Verification items for this drawing (mm, ordinates from the low corner). A direction names the side the tool comes from. Round coordinates to 2 decimals unless told otherwise and drop trailing zeros. Loops run counter-clockwise (first coordinate to the right, second up) from the corner with the lowest first, then second, coordinate; pieces in that order, holes last. Notation, with made-up numbers: M 34.25,-33 L 92.25,-33 A17 ccw 92.25,-24 Z; hole C 47,18.5 d10. An arc over 180 degrees is marked long. Use one line per item in the form item = value. Start each with the question number.
1. Draft check along Z on the marked faces 1, 2 and 3. Enter one of: pulls with the +Z half, pulls with the -Z half, needs draft (parallel to the pull), parting line crosses it, or undercut.
2. Cross-section at C-C (z = 5). Record the boundary of the cut face in (x, y).
3. Cross-section at D-D (x = 44.65). Record the boundary of the cut face in (y, z), then the cut area to 3 significant figures.
4. Go/stop test with flat-tipped pins: pin 1 (4 mm diameter, centred on x = 39, y = 20, fed in from +Z); pin 2 (10 mm diameter, centred on x = 25.5, y = 16.5, fed in from -Z); pin 3 (3 mm diameter, centred on x = 44.65, y = 15, fed in from +Z); pin 4 (2 mm diameter, centred on x = 5, z = 5, fed in from -Y). Record where each tip stops, or that it passes through.
5. Set-up check for the marked faces 4, 5 and 6: record each of +Z, -Z, +X, -X, +Y, -Y from which the full face is reachable in a straight line by a thin tool's end or side.
6. Cross-section at A-A (y = 15). Record the boundary of the cut face in (x, z), then the cut area to 3 significant figures.
7. Material ranges on line 1 (Y direction, x = 44.65, z = 48.1); line 2 (X direction, y = 3.4, z = 5); line 3 (Y direction, x = 44, z = 48), recorded low to high.
8. Cross-section at B-B (x = 53). Record the boundary of the cut face in (y, z), then the cut area to 3 significant figures.
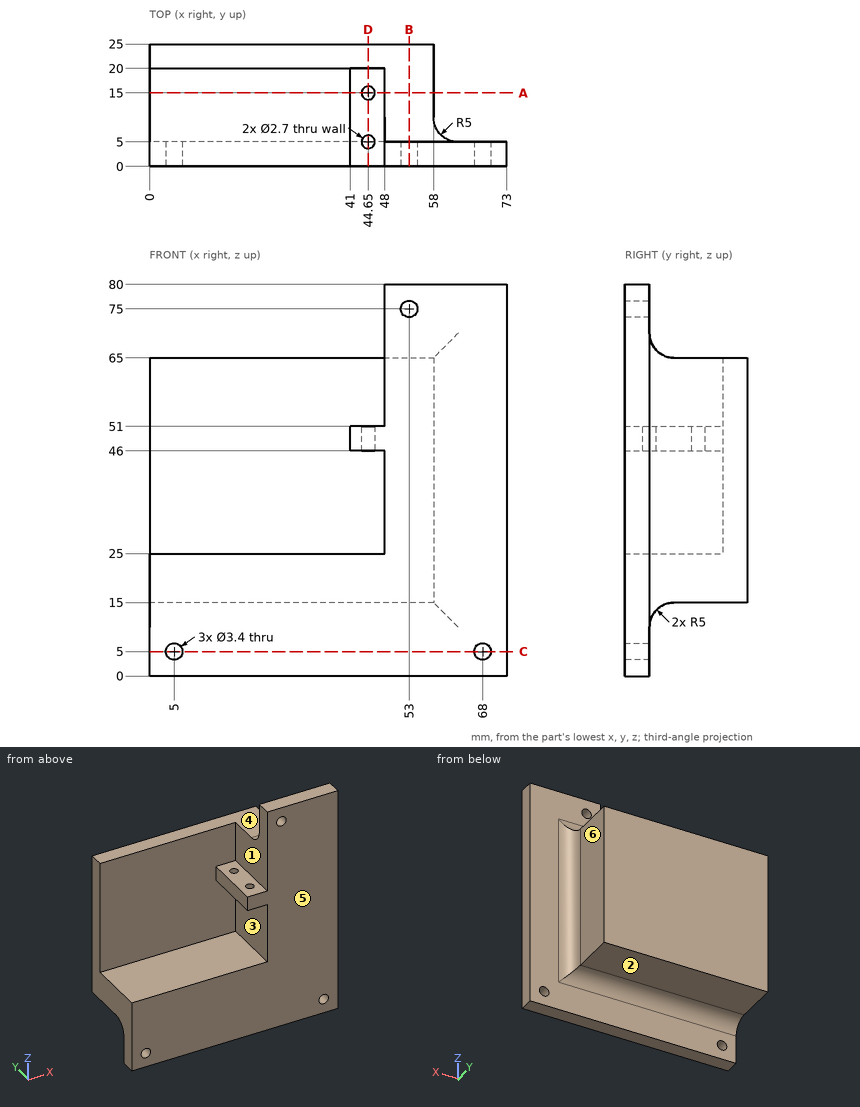
Reported:
q1.face_1 = needs draft
q1.face_2 = pulls with the -Z half
q1.face_3 = undercut
q2.outline = M 0,0 L 3.3,0 L 3.3,5 L 0,5 Z; M 6.7,0 L 66.3,0 L 66.3,5 L 6.7,5 Z; M 69.7,0 L 73,0 L 73,5 L 69.7,5 Z
q3.outline = M 0,0 L 5,0 L 5,10 A5 cw 10,15 L 25,15 L 25,65 L 20,65 L 20,51 L 16.35,51 L 16.35,46 L 20,46 L 20,25 L 0,25 Z; M 0,46 L 3.65,46 L 3.65,51 L 0,51 Z; M 6.35,46 L 13.65,46 L 13.65,51 L 6.35,51 Z
q3.area = 603 mm²
q4.pin_1 = 65
q4.pin_2 = 15
q4.pin_3 = 51
q4.pin_4 = through
q5.face_4 = +Z, +X, -X, +Y
q5.face_5 = +Z, -Z, +X, -X, -Y
q5.face_6 = +Z, -Z, +X, +Y
q6.outline = M 0,15 L 58,15 L 58,65 L 48,65 L 48,51 L 46,51 L 46,46 L 48,46 L 48,25 L 0,25 Z; M 41,46 L 43.3,46 L 43.3,51 L 41,51 Z
q6.area = 1,000 mm²
q7.line_1 = 0 to 3.65, 6.35 to 13.65, 16.35 to 25
q7.line_2 = 0 to 3.3, 6.7 to 66.3, 69.7 to 73
q7.line_3 = 0 to 3.82, 6.18 to 13.82, 16.18 to 25
q8.outline = M 0,0 L 5,0 L 5,10 A5 cw 10,15 L 25,15 L 25,65 L 10,65 A5 cw 5,70 L 5,73.3 L 0,73.3 Z; M 0,76.7 L 5,76.7 L 5,80 L 0,80 Z
q8.area = 1,390 mm²
